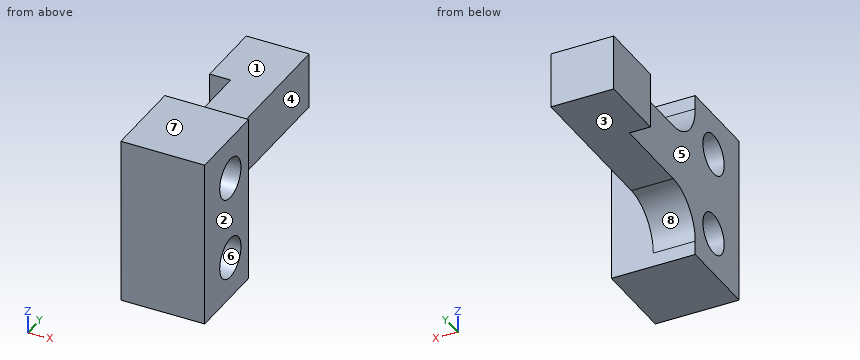
```python
from build123d import *

# Parameters (mm, degrees)
BOSS_EXTRUDE1_DEPTH    = 12
SKETCH2_W              = 4.936858862
SKETCH2_H              = 15.079572613
SKETCH2_W_2            = 5.292899171
CUT_EXTRUDE1_DEPTH     = 19.349069885
FILLET1_R              = 3
M2_5_CLEARANCE_HOLE1_D = 2.9


with BuildPart() as part:
    # Sketch1 → Boss-Extrude1 (new body)
    with BuildSketch(Plane.XY):
        Polygon((0, -6.868421053), (-6, -6.868421053), (-6, 8.131578947), (-7.5, 8.131578947), (-7.5, 13.131578947), (-3, 13.131578947), (-3, -0.868421053), (0, -0.868421053), align=None)
    extrude(amount=BOSS_EXTRUDE1_DEPTH)

    # Sketch2 → Cut-Extrude1 (cut, through all)
    with BuildSketch(Plane(origin=(-3, 0, 0), x_dir=(0, 0, -1), z_dir=(1, 0, 0))):
        with Locations((-10.468429431, 6.671365254)):
            Rectangle(SKETCH2_W, SKETCH2_H)
        with Locations((-1.353550414, 6.671365254)):
            Rectangle(SKETCH2_W_2, SKETCH2_H)
    extrude(amount=-CUT_EXTRUDE1_DEPTH, mode=Mode.SUBTRACT)

    # Fillet1
    fillet1_edges = [part.edges().sort_by_distance(p)[0] for p in [
        (-4.5, -0.868421053, 8),
        (-4.5, -0.868421053, 4),
    ]]
    fillet(fillet1_edges, radius=FILLET1_R)

    # M2.5 Clearance Hole1 (through all)
    with Locations(Plane.ZY.offset(6)):
        with Locations((3, -3.368421053), (9, -3.368421053)):
            Hole(M2_5_CLEARANCE_HOLE1_D / 2)


solid = part.part
```
CAD build for the part. Positions are in the model's coordinates, mm. Face numbers are marked on the shaded views. A direction names the side the tool comes from. Give positions to 0.01 mm unless a question says otherwise; leave off trailing zeros. Order: outer loops, then holes, each group sorted by start corner. A loop starts at its lowest first (then second) coordinate and runs counter-clockwise, first axis right, second up. Notation, with made-up numbers: M 25.25,0 L 36.25,0 A10 cw 36.25,6 Z; hole C 6,23 d4. An arc over 180 degrees is marked long. Put each result on its own line as item: value. Start each with the question number.
(1) Saw through at C-C, the plane x = -3.25. Write the cut outline in (y, z), then the cut area to 3 significant figures.
(2) Saw through at A-A, the plane z = 3. Write the cut outline in (x, y).
(3) Which spindle directions (+Z, -Z, +X, -X, +Y, -Y) get a long thin tool onto all of the face, cutting with end or side? Do the marked faces 1, 2, 3, 4 and 5. Say none if no direction does.
(4) Drill centre lines: line 1 along Y through (x, z) = (-2.5, 3); line 2 along Y through (x, z) = (-2.75, 6.5); line 3 along Z through (x, y) = (-5.75, 9.25). Where is each one in solid material? Low to high.
(5) Mould opens along Y. For the marked faces 6, 7 and 8 say: +Y half, -Y half, draft (parallel to the pull), parting line (faces both ways), or undercut.
(6) Saw through at B-B, the plane y = -2.5. Write the cut outline in (x, z).
(7) Flat gauge pins, fed straight in: pin 1 Ø1.3 at (x, y) = (-4.5, 9.5) entering from +Z; pin 2 Ø2 at (y, z) = (-1, 8.5) entering from -X; pin 3 Ø3.5 at (x, y) = (-5.5, 7.5) entering from -Z. Where does each tip first touch, or does it go through?
(8) Saw through at D-D, the plane z = 11.25. Write the cut outline in (x, y), then the cut area to 3 significant figures.
Check result:
1. outline: M -6.87,0 L -0.87,0 L -0.87,1 A3 cw 2.13,4 L 13.13,4 L 13.13,8 L 2.13,8 A3 cw -0.87,11 L -0.87,12 L -6.87,12 Z; hole C -3.37,3 d2.9; hole C -3.37,9 d2.9
1. area: 119 mm2
2. outline: M -6,-6.87 L 0,-6.87 L 0,-4.82 L -6,-4.82 Z; M -6,-1.92 L 0,-1.92 L 0,-0.87 L -3,-0.87 L -3,-0.1 L -6,-0.1 Z
3. face 1: +Z, +X, -X, +Y
3. face 2: +Z, -Z, +X, +Y, -Y
3. face 3: -Z, +X, -X, +Y
3. face 4: +Z, -Z, +X, +Y
3. face 5: +Z, -Z, -X, -Y
4. line 1: y = -6.87 to -4.82, -1.92 to -0.87
4. line 2: y = -6.87 to -0.87
4. line 3: z = 4 to 8
5. face 6: undercut
5. face 7: draft
5. face 8: +Y half
6. outline: M -6,0 L 0,0 L 0,1.84 L -6,1.84 Z; M -6,4.16 L 0,4.16 L 0,7.84 L -6,7.84 Z; M -6,10.16 L 0,10.16 L 0,12 L -6,12 Z
7. pin 1: stops at z = 8
7. pin 2: stops at x = -6
7. pin 3: stops at z = 4
8. outline: M -6,-6.87 L 0,-6.87 L 0,-0.87 L -6,-0.87 Z
8. area: 36.0 mm2
